Source: CAD feature listing. Evaluate the final solid. Frame: model axes, mm. Face numbers are marked on the shaded views. A direction names the side the tool comes from. Give positions to 0.01 mm unless a question says otherwise; leave off trailing zeros. Write each loop counter-clockwise with the first axis right and the second up, starting at its lowest first coordinate (ties: lowest second). Pieces come first, ordered by that corner, then holes. Notation, with made-up numbers: (31, -9.5) -> (37, -9.5) arc R19 cw to (37, 16.5) -> close; hole circle Ø2 at (6, 63). An arc over 180 degrees is marked (long way). Answer as a JSON object with one key per item and string values. Group by question number.
Item 1: Section query D-D on z = 6.5. Return the cut outline in (x, y), plus the area to 3 significant figures.
Item 2: Section query B-B on y = 2.5. Return the cut outline in (x, z).
Item 3: Section query A-A on x = 48. Return the cut outline in (y, z), plus the area to 3 significant figures.
Item 4: First-contact query: pin 1 Ø3 at (x, y) = (46, 3) entering from +Z; pin 2 Ø1.5 at (x, z) = (82, 4) entering from +Y; pin 3 Ø3 at (x, z) = (81, 4.5) entering from -Y; pin 4 Ø23 at (x, y) = (0, 0) entering from +Z. Flat tips, straight axial feed; report the tip coordinate or a pass-through.
Item 5: Pull-direction query (X, two-part tool) for the marked faces 1, 2 and 3; classes: pulls with the +X half, pulls with the -X half, needs draft (parallel to the pull), parting line crosses it, or undercut.
Item 6: Ray query, probe 1 along Y at (x, z) = (48, 8.25); probe 2 along Y at (x, z) = (0, 8.75); probe 3 along X at (y, z) = (-0.5, 16). Return the intervals inside material, ascending. Write a range as from..to.
Item 7: Access query for the marked faces 4, 5 and 6. Directions: +Z, -Z, +X, -X, +Y, -Y. A direction counts if a zero-diameter tool reaches every point of the face in a straight line with its end or side. Return the directions, or none.
Item 8: Section query C-C on z = 27.5. Return the cut outline in (x, y).
Autodesk Inventor part; units mm, degrees
ref_plane "YZ Plane" through (0, 0, 0) normal (1, 0, 0) x (0, 1, 0)
ref_plane "XZ Plane" through (0, 0, 0) normal (0, 1, 0) x (-1, 0, 0)
ref_plane "XY Plane" through (0, 0, 0) normal (0, 0, 1) x (1, 0, 0)
sketch "Sketch1" plane through (0, 0, 0) normal (0, 0, 1) x (1, 0, 0)
  circle A0 centre (0, 0) radius 15
  circle A1 centre (0, 0) radius 10
  circle A2 centre (0, 0) radius 30
  circle A3 centre (95.994, 1.0738) radius 10
  circle A4 centre (95.994, 1.0738) radius 20
  circle A5 centre (48, 0) radius 5
  line L0 (96, -18.9262) -> (74.477, -18.9262)
  line L1 (0, -30) -> (60, -30)
  arc A6 (74.477, -18.9262) -> (60, -30) centre (74.477, -33.9262) ccw
  line L2 (0, 30) -> (60, 30)
  line L3 (95.994, 21.0738) -> (73.7153, 21.0738)
  arc A7 (60, 30) -> (73.7153, 21.0738) centre (73.7153, 36.0738) ccw
  dimension "d0" = 30
  dimension "d1" = 20
  dimension "d2" = 60
  dimension "d6" = 20
  dimension "d7" = 40
  dimension "d8" = 10
  dimension "d9" = 48
  dimension "d10" = 96
  dimension "d11" = 60
  dimension "d12" = 30
  dimension "d13" = 60
  dimension "d14" = 30
extrude "Extrusion1" add sketch "Sketch1" along normal blind 10 contours A0 | A2 | A4 | A2 L2 A7 L3 A4 L0 A6 L1
sketch "Sketch2" plane through (0, 0, 10) normal (0, 0, 1) x (1, 0, 0)
  circle A0 centre (0, 0) radius 10
  circle A1 centre (0, 0) radius 15
  dimension "d17" = 20
  dimension "d18" = 30
extrude "Extrusion2" add sketch "Sketch2" along normal blind 20
properties part number "4-3"
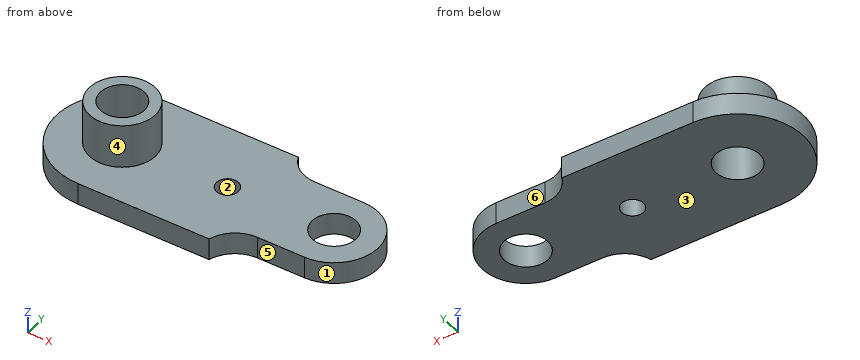
Worked answers:
{
 "1": {"outline": "(0, -30) -> (60, -30) arc R15 cw to (74.48, -18.93) -> (96, -18.93) arc R20 ccw to (95.99, 21.07) -> (73.72, 21.07) arc R15 cw to (60, 30) -> (0, 30) arc R30 ccw to start; hole circle Ø20 at (0, 0); hole circle Ø10 at (48, 0); hole circle Ø20 at (95.99, 1.07)", "area": "6,450 mm^2"},
 "2": {"outline": "(-29.9, 0) -> (-9.68, 0) -> (-9.68, 30) -> (-14.79, 30) -> (-14.79, 10) -> (-29.9, 10) -> close; (9.68, 0) -> (43.67, 0) -> (43.67, 10) -> (14.79, 10) -> (14.79, 30) -> (9.68, 30) -> close; (52.33, 0) -> (86.1, 0) -> (86.1, 10) -> (52.33, 10) -> close; (105.89, 0) -> (115.94, 0) -> (115.94, 10) -> (105.89, 10) -> close"},
 "3": {"outline": "(-30, 0) -> (-5, 0) -> (-5, 10) -> (-30, 10) -> close; (5, 0) -> (30, 0) -> (30, 10) -> (5, 10) -> close", "area": "500 mm^2"},
 "4": {"pin 1": "z = 10", "pin 2": "y = 21.07", "pin 3": "y = -18.93", "pin 4": "z = 30"},
 "5": {"face 1": "pulls with the +X half", "face 2": "undercut", "face 3": "needs draft"},
 "6": {"probe 1": "-30..-5, 5..30", "probe 2": "-30..-10, 10..30", "probe 3": "-14.99..-9.99, 9.99..14.99"},
 "7": {"face 4": "+Z", "face 5": "+Z, -Z, +X, -Y", "face 6": "+Z, -Z, +X, +Y"},
 "8": {"outline": "circle Ø30 at (0, 0); hole circle Ø20 at (0, 0)"}
}
